Read the model definition and answer for the solid it produces. Units are mm, in the model's axes. Give positions to 0.01 mm unless a question says otherwise; leave off trailing zeros. Write each loop counter-clockwise with the first axis right and the second up, starting at its lowest first coordinate (ties: lowest second). Pieces come first, ordered by that corner, then holes. Notation, with made-up numbers: M 25.25,88.5 L 46.25,88.5 A32 ccw 46.25,125.5 Z; hole C 22,77 d1. An arc over 180 degrees is marked long. Answer as CSV lines item,"result". Start each with the question number.
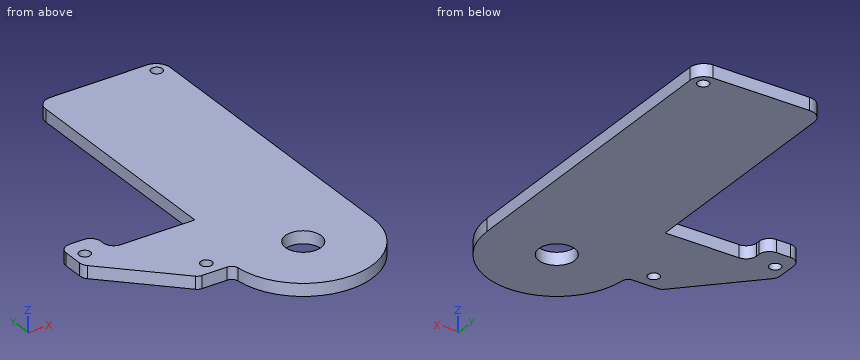
Autodesk Inventor part; units mm, degrees
ref_plane "YZ Plane" through (0, 0, 0) normal (1, 0, 0) x (0, 1, 0)
ref_plane "XZ Plane" through (0, 0, 0) normal (0, 1, 0) x (-1, 0, 0)
ref_plane "XY Plane" through (0, 0, 0) normal (0, 0, 1) x (1, 0, 0)
sketch "Sketch1" plane through (0, 0, 0) normal (0, 0, 1) x (1, 0, 0)
  circle A0 centre (25.0558, -45.1154) radius 20
  line L0 (45.0558, -45.1154) -> (31.0558, -45.1154)
  line L1 (31.0558, -45.1154) -> (31.0558, -22.1154)
  line L2 (31.0558, -22.1154) -> (45.0558, -22.1154)
  line L3 (45.0558, -22.1154) -> (45.0558, -45.1154)
  line L4 (31.0558, -22.1154) -> (-4.9442, -22.1154)
  line L5 (-4.9442, -22.1154) -> (-4.9442, -45.1154)
  line L6 (-4.9442, -45.1154) -> (31.0558, -45.1154)
  line L7 (31.0558, -45.1154) -> (31.0558, -22.1154)
  line L8 (-4.9442, -45.1154) -> (-24.9442, -25.1154)
  line L9 (-24.9442, -25.1154) -> (-24.9442, -15.1154)
  line L10 (-24.9442, -15.1154) -> (-4.9442, -15.1154)
  line L11 (-4.9442, -15.1154) -> (-4.9442, -22.1154)
  point P0 (0, 0)
  dimension "d0" = 40
  dimension "d1" = 14
  dimension "d2" = 23
  dimension "d20" = 0
  dimension "d21" = 23
  dimension "d22" = 30
  dimension "d23" = 20
  dimension "d24" = 50
  dimension "d45" = 10
extrude "Extrusion1" add sketch "Sketch1" along normal blind 3.6
sketch "Sketch2" plane through (0, 0, 3.6) normal (0, 0, 1) x (1, 0, 0)
  arc A0 (5.0558, -45.1154) -> (45.0558, -45.1154) centre (25.0558, -45.1154) ccw
  circle A1 centre (25.0558, -45.1154) radius 5.15
  circle A2 centre (0.0558, -40.8364) radius 1.625
  line L0 (-4.9442, -22.1154) -> (-4.9442, -45.1154)
  line L1 (-4.9442, -45.1154) -> (5.0558, -45.1154)
  line L2 (45.0558, -45.1154) -> (45.0558, -22.1154)
  line L3 (45.0558, -22.1154) -> (-4.9442, -22.1154)
  circle A3 centre (-21.4442, -20.8364) radius 1.625
  point P0 (0, 0)
  point P1 (30.9974, -15.1154)
  dimension "d5" = 10.3
  dimension "d6" = 3.25
  dimension "d10" = 4.279
  dimension "d18" = 23
  dimension "d25" = 3.25
  dimension "d26" = 20
  dimension "d27" = 21.5
extrude "Extrusion2" cut sketch "Sketch2" against normal blind 20 contours A1 | A2 | A3
fillet "Fillet1" radius 2 4 edges at (45.0558, -22.1154, 1.8) (-4.9442, -45.1154, 1.8) (-4.9442, -22.1154, 1.8) (5.0558, -45.1154, 1.8)
fillet "Fillet2" radius 3 3 edges at (-24.9442, -25.1154, 1.8) (-24.9442, -15.1154, 1.8) (-4.9442, -15.1154, 1.8)
sketch "Sketch3" plane through (0, 0, 0) normal (0, 0, -1) x (-1, 0, 0)
  line L0 (7.9442, -15.1154) -> (21.9442, -15.1154)
  line L1 (14.9442, -15.1154) -> (-0.0558, -15.1154)
  line L2 (-0.0558, -15.1154) -> (-0.0558, -22.1154)
  line L3 (-0.0558, -22.1154) -> (14.9442, -22.1154)
  line L4 (14.9442, -22.1154) -> (14.9442, -15.1154)
  line L5 (4.9442, -19.1154) -> (4.9442, -18.1154)
  point P0 (0, 0)
  dimension "d29" = 7
  dimension "d32" = 15
  dimension "d33" = 5
extrude "Extrusion3" cut sketch "Sketch3" against normal blind 10
fillet "Fillet3" radius 3 2 edges at (-14.9442, -15.1154, 1.8) (-14.9442, -22.1154, 1.8)
sketch "Sketch4" plane through (0, 0, 0) normal (0, 0, -1) x (-1, 0, 0)
  line L0 (-45.0558, -45.1154) -> (-45.0558, -24.1154)
  line L1 (-45.0558, -28.8196) -> (-9.3289, -28.8196)
  line L2 (-9.3289, -28.8196) -> (-9.3289, 45.6636)
  line L3 (-9.3289, 45.6636) -> (-45.0558, 45.6636)
  line L4 (-45.0558, 45.6636) -> (-45.0558, -28.8196)
  line L5 (-43.0558, -22.1154) -> (11.9442, -22.1154)
  circle A0 centre (-0.0558, -40.8364) radius 1.625
  point P0 (0, 0)
  dimension "d36" = 86.5
extrude "Extrusion4" add sketch "Sketch4" against normal blind 3.6 contours L0 L4 L3 L2 L1
fillet "Fillet4" radius 4 2 edges at (9.3289, 45.6636, 1.8) (45.0558, 45.6636, 1.8)
sketch "Sketch5" plane through (0, 0, 0) normal (0, 0, -1) x (-1, 0, 0)
  circle A0 centre (-41.5558, 42.1636) radius 1.625
  line L0 (-13.3289, 45.6636) -> (-41.0558, 45.6636)
  line L1 (-45.0558, 41.6636) -> (-45.0558, -45.1154)
  point P0 (0, 0)
  point P1 (-41.0558, 41.6636)
  dimension "d40" = 3.25
  dimension "d43" = 3.5
  dimension "d44" = 3.5
extrude "Extrusion5" cut sketch "Sketch5" against normal blind 5
properties part number "p6"
1. Find the intervals of material crossed by line 1 (Y direction, x = 25.5, z = 3.3); line 2 (X direction, y = 26, z = 1.5); line 3 (Y direction, x = -2, z = 0.8), in increasing order. Write a range as [from, to].
2. Find section A-A on z = 1.3. Determine the outline of the cut face in (x, y) (3 decimals), then the cut area to 3 significant figures.
3. Find section B-B on y = 1. Determine the outline of the cut face in (x, z).
4. Find section C-C on x = -13. Determine the outline of the cut face in (y, z).
5. Given pin 1 (13.5 mm diameter, centred on x = 25.06, y = -45.12, fed in from +Z); pin 2 (1.9 mm diameter, centred on x = 41.56, y = 42.16, fed in from +Z); pin 3 (1.1 mm diameter, centred on x = 1.5, z = 2, fed in from +Y); pin 4 (1.8 mm diameter, centred on y = -5, z = 2, fed in from -X), each flat-ended and moving along its own axis, determine where each tip first touches the part or whether it passes through.
Computed:
1,line 1,"y = [-65.11, -50.25], [-39.98, 45.66]"
1,line 2,"x = [9.33, 45.06]"
1,line 3,"y = [-45.12, -22.12]"
2,outline,"M -24.944,-23.873 A3 ccw -24.066,-25.994 L -5.53,-44.53 A2 ccw -4.116,-45.115 L 3.147,-45.115 A2 cw 5.139,-46.934 A20 ccw 45.056,-45.115 L 45.056,41.664 A4 ccw 41.056,45.664 L 13.329,45.664 A4 ccw 9.329,41.664 L 9.329,-22.115 L -11.944,-22.115 A3 cw -14.944,-19.115 L -14.944,-18.115 A3 ccw -17.944,-15.115 L -21.944,-15.115 A3 ccw -24.944,-18.115 Z; hole C -21.444,-20.836 d3.25; hole C 0.056,-40.836 d3.25; hole C 25.056,-45.115 d10.3; hole C 41.556,42.164 d3.25"
2,area,"4,410 mm^2"
3,outline,"M 9.33,0 L 45.06,0 L 45.06,3.6 L 9.33,3.6 Z"
4,outline,"M -37.06,0 L -21.92,0 L -21.92,3.6 L -37.06,3.6 Z"
5,pin 1,"stops at z = 3.6"
5,pin 2,"passes through"
5,pin 3,"stops at y = -22.12"
5,pin 4,"stops at x = 9.33"
